Design review of the part built by this model. Coordinates are the model's own, in mm. Coordinates: 2 decimals unless noted, no trailing zeros. Write each loop counter-clockwise with the first axis right and the second up, starting at its lowest first coordinate (ties: lowest second). Pieces come first, ordered by that corner, then holes. Notation, with made-up numbers: M 36,77.25 L 40,77.25 A23 cw 40,105.25 Z; hole C 0.25,66 d8. An arc over 180 degrees is marked long. Write item = value, one per line.
```python
from build123d import *

# Parameters (mm, degrees)
F0_R     = 6
F0_R_2   = 0.5
F1_DEPTH = 4
F2_R     = 0.5


with BuildPart() as f1:
    # F0 (on Right) → F1 (new body)
    with BuildSketch(Plane.YZ):
        Circle(F0_R)
        with Locations((0, -2)):
            Circle(F0_R_2, mode=Mode.SUBTRACT)
        with Locations((-2, 0)):
            Circle(F0_R_2, mode=Mode.SUBTRACT)
        with Locations((2, 0)):
            Circle(F0_R_2, mode=Mode.SUBTRACT)
        with Locations((0, 2)):
            Circle(F0_R_2, mode=Mode.SUBTRACT)
    extrude(amount=F1_DEPTH)

    # F2
    f2_edges = [f1.edges().sort_by_distance(p)[0] for p in [
        (4, -6, 0),
        (0, -6, 0),
    ]]
    fillet(f2_edges, radius=F2_R)


solid = f1.part
```
Q1. Wall thickness on line 1 (Z direction, x = 3, y = 0); line 2 (Y direction, x = 0.95, z = 1.75); line 3 (Z direction, x = 1.65, y = 2): over which ranges is each line inside the solid? List them lowest first.
Check result:
line_1 = -6 to -2.5, -1.5 to 1.5, 2.5 to 6
line_2 = -5.74 to -0.43, 0.43 to 5.74
line_3 = -5.66 to -0.5, 0.5 to 5.66
Q2. Consider section A-A, the plane y = 0. State the section outline as (x, z) points, and give its area (3 significant figures).
Check result:
outline = M 0,-5.5 A0.5 ccw 0.5,-6 L 3.5,-6 A0.5 ccw 4,-5.5 L 4,-2.5 L 0,-2.5 Z; M 0,-1.5 L 4,-1.5 L 4,1.5 L 0,1.5 Z; M 0,2.5 L 4,2.5 L 4,5.5 A0.5 ccw 3.5,6 L 0.5,6 A0.5 ccw 0,5.5 Z
area = 39.8 mm²
Q3. For P1, Ø1, axis at x = 2, y = 3, coming from the +Z side; P2, Ø1, axis at x = 2, z = -1.5, coming from the +Y side, all flat-tipped, find the tip position at first contact; note any pin that passes through.
Check result:
P1 = 5.45
P2 = 5.92
Q4. Consider section C-C, the plane x = 2.7. State the section outline as (y, z) points, and give its area (3 significant figures).
Check result:
outline = C 0,0 d12; hole C -2,0 d1; hole C 0,-2 d1; hole C 0,2 d1; hole C 2,0 d1
area = 110 mm²
Q5. The part is to be moulded in two halves that separate along Z. For faces 1 (the flat face through (4, 0, 0)), 2 (the cylindrical face through (2, -6, 0)), 3 (the cylindrical face through (2, -2.4, -0.3)), 4 (the cylindrical face through (1.972, -0.065, -1.504)), say which applies: +Z half, -Z half, draft (parallel to the pull), parting line (faces both ways), or undercut.
Check result:
face_1 = draft
face_2 = parting line
face_3 = undercut
face_4 = undercut
